Can you work these out from the model? Positions are in its coordinate system, mm. Face numbers are marked on the shaded views. A direction names the side the tool comes from. Round coordinates to 2 decimals unless told otherwise and drop trailing zeros. Order: outer loops, then holes, each group sorted by start corner. A loop starts at its lowest first (then second) coordinate and runs counter-clockwise, first axis right, second up.
from build123d import *

# Parameters (mm, degrees)
F3_DEPTH = 20
F4_R     = 4.99999
F6_DEPTH = 2.6
F7_D     = 3.6
F7_DEPTH = 10
F7_TIP   = 1.0815491142
F8_R     = 40


# Not quite as in the source:
# - a fillet or chamfer is up to 0.001 mm smaller than in the source, because OpenCascade refuses the exact size


with BuildPart() as f3:
    # F2 (on Top) → F3 (new body)
    with BuildSketch(Plane.XY):
        Polygon((0, 5), (0, 0), (20, 0), (20, -34), (0, -34), (0, -39), (30, -39), (30, 0), (80, 0), (80, 15), (75, 15), (75, 5), align=None)
    extrude(amount=F3_DEPTH)

    # F4 (radius 5 in the source; OpenCascade refuses exactly that, so slightly less here)
    f4_edges = [f3.edges().sort_by_distance(p)[0] for p in [
        (30, -39, 10),
        (80, 0, 10),
        (80, 15, 10),
        (0, 5, 10),
        (0, -39, 10),
    ]]
    fillet(f4_edges, radius=F4_R)

    # F5 (on face) → F6 (cut)
    with BuildSketch(Plane(origin=(0, -34, 0), x_dir=(-1, 0, 0), z_dir=(0, 1, 0))):
        Polygon((-7.25, 8.4122867597), (-7.25, 11.5877132403), (-10, 13.1754264805), (-12.75, 11.5877132403), (-12.75, 8.4122867597), (-10, 6.8245735195), align=None)
    extrude(amount=-F6_DEPTH, mode=Mode.SUBTRACT)

    # F7 (one way)
    with BuildSketch(Plane(origin=(0, -34, 0), x_dir=(-1, 0, 0), z_dir=(0, 1, 0))):
        with Locations((-10, 10)):
            Circle(F7_D / 2)
    extrude(amount=-F7_DEPTH, mode=Mode.SUBTRACT)
    with Locations(Plane(origin=(0, -34, 0), x_dir=(-1, 0, 0), z_dir=(0, 1, 0))):
        with Locations((-10, 10)):
            with Locations((0, 0, -(F7_DEPTH + F7_TIP / 2))):  # 118° drill point
                Cone(0, F7_D / 2, F7_TIP, mode=Mode.SUBTRACT)

    # F8
    f8_edges = [f3.edges().sort_by_distance(p)[0] for p in [
        (30, 0, 10),
    ]]
    fillet(f8_edges, radius=F8_R)


solid = f3.part
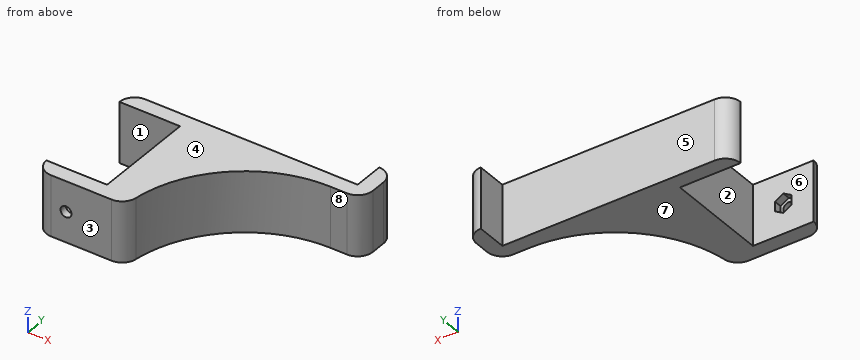
(1) I'm going to push flat-ended pins straight in: pin 1 Ø10 at (x, z) = (53.5, 7.5) entering from +Y; pin 2 Ø1.3 at (y, z) = (-36, 9.5) entering from +X; pin 3 Ø6 at (x, z) = (72.5, 8) entering from -Y. Where does each tip first touch, or does it pass through?
(2) Please list where these lines run through material, in increasing order: probe 1 along Y at (x, z) = (17, 15.75); probe 2 along Z at (x, y) = (10, -38); probe 3 along Y at (x, z) = (69, 3.75).
(3) If we mould it in two halves opening along Y, with no side actions, what happens to the marked faces 1, 2, 3 and 4? For each: pulls with the +Y half, pulls with the -Y half, needs draft (parallel to the pull), parting line crosses it, or undercut.
(4) I want a section at B-B, the plane x = 26.5. List the corners of the cut face in (y, z) for me, plus the area to 3 significant figures.
(5) I want a section at A-A, the plane x = 6. List the corners of the cut face in (y, z) for me, plus the area to 3 significant figures.
(6) On a 3-axis mill with a long thin cutter (end or side, diameter ignored), from which of +Z, -Z, +X, -X, +Y, -Y can I reach the whole of each face in a straight line? I mean the marked faces 5, 6, 7 and 8. Say none if no direction works.
Ans:
1. pin 1: stops at y = 5
1. pin 2: stops at x = 29.81
1. pin 3: stops at y = 0
2. probe 1: y = -39 to -34, 0 to 5
2. probe 2: z = 0 to 8.2, 11.8 to 20
2. probe 3: y = 0 to 5
3. face 1: undercut
3. face 2: undercut
3. face 3: pulls with the -Y half
3. face 4: needs draft
4. outline: (-38.77, 0) - (5, 0) - (5, 20) - (-38.77, 20) - close
4. area: 875 mm2
5. outline: (-39, 0) - (-34, 0) - (-34, 20) - (-39, 20) - close; (0, 0) - (5, 0) - (5, 20) - (0, 20) - close
5. area: 200 mm2
6. face 5: +Z, -Z, -X, +Y
6. face 6: +Z, -Z, -X
6. face 7: -Z, +X, -X, +Y, -Y
6. face 8: +Z, -Z, +X, -Y
